Verification items for the finished model (mm, model axes). A direction names the side the tool comes from. Give positions to 0.01 mm unless a question says otherwise; leave off trailing zeros. Loops run counter-clockwise (first coordinate to the right, second up) from the corner with the lowest first, then second, coordinate; pieces in that order, holes last. Notation, with made-up numbers: (-13, -16) -> (3, -16) arc R21 ccw to (3, -9) -> close; hole circle Ø2 at (46, 58.5). An arc over 180 degrees is marked (long way). Answer in a Markdown table with one row per item. Add a question column.
Q1. Material ranges on probe 1 along X at (y, z) = (10.75, 0); probe 2 along X at (y, z) = (8, 4); probe 3 along X at (y, z) = (17.5, -28.5), recorded low to high.
Q2. Section check B-B on x = 0. Enter the section's corners in (y, z), and give its area (3 significant figures).
Q3. Gauge pin test, flat ends, axial feed: P1, Ø8.5, axis at x = -27.75, z = 0, coming from the +Y side; P2, Ø1, axis at x = -27, y = 16, coming from the -Z side; P3, Ø3, axis at x = 12.5, y = 14, coming from the +Z side. Record the tip position at first contact, or that the pin passes through.
Q4. Release check for a two-part mould opening along X. For faces 1 (the face through (-42.594, 9.86, -55.55)), 2 (the face through (-15, 0, 15)), 3 (the face through (-7.1, 13.7, 21.9)) record: pulls with the +X half, pulls with the -X half, needs draft (parallel to the pull), parting line crosses it, or undercut.
Q5. Section check D-D on x = -32.5. Enter the section's corners in (y, z), and give its area (3 significant figures).
Q6. Section check C-C on y = 12.75. Enter the section's corners in (x, z), and give its area (3 significant figures).
Q7. Section check A-A on z = 0. Enter the section's corners in (x, y), and give its area (3 significant figures).
Q8. Set-up check for faces 4 (the face through (12.95, 13.73, -31.08)), 5 (the face through (-19.524, 9.86, -4.336)): record each of +Z, -Z, +X, -X, +Y, -Y from which the full face is reachable in a straight line by a thin tool's end or side.
```python
from build123d import *

# Parameters (mm, degrees)
SKETCH1_R             = 70
BOSS_EXTRUDE1_DEPTH   = 20
SKETCH2_R             = 20
CUT_EXTRUDE1_DEPTH    = 101.995049384
SKETCH3_R             = 7.105797858
CUT_EXTRUDE2_DEPTH    = 12.372306
CIRPATTERN1_START     = 7.627693822
CIRPATTERN1_OUTLINE_R = 7.105797858
CIRPATTERN1_DEPTH     = 12.372306178


# Read off the part's stored shape, not the designer's step: CirPattern1
with BuildPart() as part:
    # Sketch1 → Boss-Extrude1 (new body)
    with BuildSketch(Plane(origin=(0, 0, 0), x_dir=(1, 0, 0), z_dir=(0, 1, 0))):
        with Locations(Location((0, 0, 0), (0, 0, 270))):
            Circle(SKETCH1_R)
    extrude(amount=BOSS_EXTRUDE1_DEPTH)

    # Sketch2 → Cut-Extrude1 (cut, through all)
    with BuildSketch(Plane(origin=(0, 0, 0), x_dir=(1, 0, 0), z_dir=(0, 1, 0))):
        with Locations(Location((0, 0, 0), (0, 0, 270))):
            Circle(SKETCH2_R)
    extrude(amount=CUT_EXTRUDE1_DEPTH, mode=Mode.SUBTRACT)

    # Sketch3 → Cut-Extrude2 (cut)
    with BuildSketch(Plane(origin=(0, 20, 0), x_dir=(1, 0, 0), z_dir=(0, 1, 0))):
        with Locations(Location((-27.753811795, 0, 0), (0, 0, 270))):
            Circle(SKETCH3_R)
    extrude(amount=-CUT_EXTRUDE2_DEPTH, mode=Mode.SUBTRACT)

    # CirPattern1 outline → CirPattern1 (cut)
    with BuildSketch(Plane(origin=(0, 0, 0), x_dir=(1, 0, 0), z_dir=(0, 1, 0)).offset(CIRPATTERN1_START)):
        with Locations((-13.876905897, -24.035506066)):
            Circle(CIRPATTERN1_OUTLINE_R)
        with Locations((13.876905897, -24.035506066)):
            Circle(CIRPATTERN1_OUTLINE_R)
        with Locations((27.753811795, 0)):
            Circle(CIRPATTERN1_OUTLINE_R)
        with Locations((13.876905897, 24.035506066)):
            Circle(CIRPATTERN1_OUTLINE_R)
        with Locations((-13.876905897, 24.035506066)):
            Circle(CIRPATTERN1_OUTLINE_R)
    extrude(amount=CIRPATTERN1_DEPTH, mode=Mode.SUBTRACT)


solid = part.part
```
Taken from the geometry:
| question | item | result |
|---|---|---|
| 1 | probe 1 | x = -70 to -34.86, -20.65 to -20, 20 to 20.65, 34.86 to 70 |
| 1 | probe 2 | x = -69.89 to -33.63, -21.88 to -19.6, 19.6 to 21.88, 33.63 to 69.89 |
| 1 | probe 3 | x = -63.94 to -19.41, -8.35 to 8.35, 19.41 to 63.94 |
| 2 | outline | (0, -70) -> (20, -70) -> (20, -20) -> (0, -20) -> close; (0, 20) -> (20, 20) -> (20, 70) -> (0, 70) -> close |
| 2 | area | 2,000 mm² |
| 3 | P1 | stops at y = 7.63 |
| 3 | P2 | stops at z = -64.79 |
| 3 | P3 | stops at z = 69.13 |
| 4 | face 1 | parting line crosses it |
| 4 | face 2 | needs draft |
| 4 | face 3 | undercut |
| 5 | outline | (0, -62) -> (20, -62) -> (20, -5.29) -> (7.63, -5.29) -> (7.63, 5.29) -> (20, 5.29) -> (20, 62) -> (0, 62) -> close |
| 5 | area | 2,350 mm² |
| 6 | outline | circle Ø140 at (0, 0); hole circle Ø14.21 at (-27.75, 0); hole circle Ø14.21 at (-13.88, -24.04); hole circle Ø14.21 at (-13.88, 24.04); hole circle Ø40 at (0, 0); hole circle Ø14.21 at (13.88, -24.04); hole circle Ø14.21 at (13.88, 24.04); hole circle Ø14.21 at (27.75, 0) |
| 6 | area | 13,200 mm² |
| 7 | outline | (-70, 0) -> (-20, 0) -> (-20, 20) -> (-20.65, 20) -> (-20.65, 7.63) -> (-34.86, 7.63) -> (-34.86, 20) -> (-70, 20) -> close; (20, 0) -> (70, 0) -> (70, 20) -> (34.86, 20) -> (34.86, 7.63) -> (20.65, 7.63) -> (20.65, 20) -> (20, 20) -> close |
| 7 | area | 1,650 mm² |
| 8 | face 4 | +Y |
| 8 | face 5 | +Y, -Y |
